```python
from build123d import *
from build123d.topology import SkipClean

# Parameters (mm, degrees)
SKETCH_1_R             = 43
SKETCH_1_R_2           = 1.75
EXTRUDE_1_DEPTH        = 3
EXTRUDE_1_2_DEPTH      = 19
EXTRUDE_1_2_DEPTH_BACK = 33
SKETCH_3_R             = 43
SKETCH_3_R_2           = 40.5
EXTRUDE_START          = -52
EXTRUDE_2_DEPTH        = 52
EXTRUDE_2_2_DEPTH      = 2.5
FILLET_1_R             = 2
SKETCH_6_W             = 12.068691
SKETCH_6_H             = 10.532676
CUT_EXTRUDE_1_DEPTH    = 3
SKETCH_7_R             = 2
CUT_EXTRUDE_2_DEPTH    = 283
SKETCH_8_R             = 2
CUT_EXTRUDE_3_DEPTH    = 10
SKETCH_9_W             = 13.11693
SKETCH_9_H             = 19.719399
CUT_EXTRUDE_4_DEPTH    = 10
SKETCH_10_W            = 7.55958
SKETCH_10_H            = 12.395118
CUT_EXTRUDE_5_DEPTH    = 61
SKETCH_11_W            = 11.880057
SKETCH_11_H            = 21.859304
CUT_EXTRUDE_6_DEPTH    = 61
SKETCH_12_R            = 4.8
CUT_EXTRUDE_7_DEPTH    = 10
SKETCH_13_R            = 4.906551
CUT_EXTRUDE_8_DEPTH    = 10


with BuildPart() as part:
    # 草图1 → Extrude 1 (new body)
    with BuildSketch(Plane.XY):
        with Locations((0, 10.35)):
            Circle(SKETCH_1_R)
        with Locations((-5, 24.315)):
            Circle(SKETCH_1_R_2, mode=Mode.SUBTRACT)
        with Locations((5, 24.315)):
            Circle(SKETCH_1_R_2, mode=Mode.SUBTRACT)
        with Locations((-5, -24.315)):
            Circle(SKETCH_1_R_2, mode=Mode.SUBTRACT)
        with Locations((5, -24.315)):
            Circle(SKETCH_1_R_2, mode=Mode.SUBTRACT)
        with BuildLine():
            Line((3.395324, 20.5), (10.5, 20.5))
            Line((10.5, 20.5), (10.5, -20.5))
            Line((10.5, -20.5), (-10.5, -20.5))
            Line((-10.5, -20.5), (-10.5, 20.5))
            Line((-10.5, 20.5), (-3.395324, 20.5))
            ThreePointArc((-3.395324, 20.5), (0, 23.895324), (3.395324, 20.5))
        make_face(mode=Mode.SUBTRACT)
        with BuildLine():
            Line((-14.5, 48.165341), (-14.5, -27.465341))
            ThreePointArc((-14.5, -27.465341), (-40.5, 10.35), (-14.5, 48.165341))
        make_face(mode=Mode.SUBTRACT)
        with BuildLine():
            Line((14.5, 48.165341), (14.5, -27.465341))
            ThreePointArc((14.5, -27.465341), (40.5, 10.35), (14.5, 48.165341))
        make_face(mode=Mode.SUBTRACT)
    extrude(amount=EXTRUDE_1_DEPTH)

    # 草图3 → Extrude 1 2 (add, two sides: drawn at the far end of the back side and taken through both)
    with SkipClean():  # the faces are left unmerged after this step: merging them gives an invalid solid
        with BuildSketch(Plane(origin=(0, 0, 0), x_dir=(-1, 0, 0), z_dir=(0, 0, -1)).offset(-EXTRUDE_1_2_DEPTH_BACK)):
            with Locations((0, 10.35)):
                Circle(SKETCH_3_R)
            with Locations((0, 10.35)):
                Circle(SKETCH_3_R_2, mode=Mode.SUBTRACT)
        extrude(amount=EXTRUDE_1_2_DEPTH + EXTRUDE_1_2_DEPTH_BACK)

    # 草图4 → Extrude 2 (add)
    with SkipClean():  # the faces are left unmerged after this step: merging them gives an invalid solid
        with BuildSketch(Plane(origin=(0, 0, -19), x_dir=(-1, 0, 0), z_dir=(0, 0, -1)).offset(EXTRUDE_START)):
            Polygon((0, 53.35), (210, 53.35), (210, -243.65), (0, -243.65), (0, -30.15), (2.5, -30.15), (2.5, -241.15), (207.5, -241.15), (207.5, 50.85), (0, 50.85), align=None)
        extrude(amount=EXTRUDE_2_DEPTH)

    # 草图5 → Extrude 2 2 (add)
    with SkipClean():  # the faces are left unmerged after this step: merging them gives an invalid solid
        with BuildSketch(Plane(origin=(0, 0, -19), x_dir=(-1, 0, 0), z_dir=(0, 0, -1))):
            with BuildLine():
                Line((2.5, -241.15), (2.5, -32.577264))
                ThreePointArc((2.5, -32.577264), (42.565682, 4.25388), (14.448183, 50.85))
                Line((14.448183, 50.85), (207.5, 50.85))
                Line((207.5, 50.85), (207.5, -241.15))
                Line((207.5, -241.15), (2.5, -241.15))
            make_face()
        extrude(amount=-EXTRUDE_2_2_DEPTH)

    # 圆角1
    fillet_1_edges = [part.edges().sort_by_distance(p)[0] for p in [
        (-207.5, 50.85, 8.25),
        (0, -243.65, 7),
        (-207.5, -241.15, 8.25),
        (-2.5, -241.15, 8.25),
        (-210, -243.65, 7),
        (-210, 53.35, 7),
    ]]
    fillet(fillet_1_edges, radius=FILLET_1_R)

    # 草图6 → 切除-拉伸1 (cut)
    with BuildSketch(Plane(origin=(0, 53.35, 0), x_dir=(1, 0, 0), z_dir=(0, 1, 0))):
        with Locations((-27.994546, 8.375655)):
            Rectangle(SKETCH_6_W, SKETCH_6_H)
    extrude(amount=-CUT_EXTRUDE_1_DEPTH, mode=Mode.SUBTRACT)

    # 草图7 → 切除-拉伸2 (cut)
    with BuildSketch(Plane(origin=(0, 0, 0), x_dir=(0, 0, -1), z_dir=(1, 0, 0))):
        with Locations(Location((-25.5, -84.801057, 0), (0, 0, 270))):
            Circle(SKETCH_7_R)
        with Locations(Location((-25.5, -190.350496, 0), (0, 0, 270))):
            Circle(SKETCH_7_R)
    extrude(amount=-CUT_EXTRUDE_2_DEPTH, mode=Mode.SUBTRACT)

    # 草图8 → 切除-拉伸3 (cut)
    with BuildSketch(Plane.XZ.offset(243.65)):
        with Locations(Location((-167.807889, 25.5, 0), (0, 0, 270))):
            Circle(SKETCH_8_R)
        with Locations(Location((-42.192111, 25.5, 0), (0, 0, 270))):
            Circle(SKETCH_8_R)
    extrude(amount=-CUT_EXTRUDE_3_DEPTH, mode=Mode.SUBTRACT)

    # 草图9 → 切除-拉伸4 (cut)
    with BuildSketch(Plane(origin=(0, 53.35, 0), x_dir=(1, 0, 0), z_dir=(0, 1, 0))):
        with Locations((-112.297275, -25.832317)):
            Rectangle(SKETCH_9_W, SKETCH_9_H)
        with BuildLine():
            Line((-92.210137, -34.22374), (-82.740067, -34.22374))
            Line((-82.740067, -34.22374), (-82.740067, -18.619532))
            ThreePointArc((-82.740067, -18.619532), (-87.475102, -14.502019), (-92.210137, -18.619532))
            Line((-92.210137, -18.619532), (-92.210137, -34.22374))
        make_face()
    extrude(amount=-CUT_EXTRUDE_4_DEPTH, mode=Mode.SUBTRACT)

    # 草图10 → 切除-拉伸5 (cut)
    with BuildSketch(Plane.ZY.offset(2.5)):
        with Locations((29.22021, 11.568763)):
            Rectangle(SKETCH_10_W, SKETCH_10_H)
    extrude(amount=CUT_EXTRUDE_5_DEPTH, mode=Mode.SUBTRACT)

    # 草图11 → 切除-拉伸6 (cut)
    with BuildSketch(Plane(origin=(0, 0, -19), x_dir=(-1, 0, 0), z_dir=(0, 0, -1))):
        with Locations((93.214773, 23.896012)):
            Rectangle(SKETCH_11_W, SKETCH_11_H)
    extrude(amount=-CUT_EXTRUDE_6_DEPTH, mode=Mode.SUBTRACT)

    # 草图12 → 切除-拉伸7 (cut)
    with BuildSketch(Plane(origin=(0, 53.35, 0), x_dir=(1, 0, 0), z_dir=(0, 1, 0))):
        with Locations(Location((-104, 6.738484, 0), (0, 0, 270))):
            Circle(SKETCH_12_R)
    extrude(amount=-CUT_EXTRUDE_7_DEPTH, mode=Mode.SUBTRACT)

    # 草图13 → 切除-拉伸8 (cut)
    with BuildSketch(Plane(origin=(0, 53.35, 0), x_dir=(1, 0, 0), z_dir=(0, 1, 0))):
        with Locations((-68.22173, -33)):
            Circle(SKETCH_13_R)
    extrude(amount=-CUT_EXTRUDE_8_DEPTH, mode=Mode.SUBTRACT)


solid = part.part
```
Work out the finished part from the listing and answer in its coordinate system (mm). A direction names the side the tool comes from. Round coordinates to 2 decimals unless told otherwise and drop trailing zeros. Loops run counter-clockwise (first coordinate to the right, second up) from the corner with the lowest first, then second, coordinate; pieces in that order, holes last. Notation, with made-up numbers: M -32.5,40 L -12.5,40 A26 ccw -12.5,72 Z; hole C -4,78 d8. An arc over 180 degrees is marked long. One line per question, with ' | ' between items.
Q1. A tool of negligible diameter and unlimited length cuts with its end or side. For faces 1 (the flat face through (0, -139, 7)), 2 (the flat face through (-106, -93, -16.5)), 3 (the flat face through (0, 29, 0)), 4 (the flat face through (-106, -243.65, 7)), from which of +Z, -Z, +X, -X, +Y, -Y can it reach the whole face along a straight path? Write none if from no direction.
Conclusion:
face 1: +Z, -Z, +X, -Y | face 2: +Z | face 3: -Z | face 4: +Z, -Z, +X, -X, -Y
Q2. The mould has two halves that part along Z. Classify faces 5 (the flat face through (0, 29, 3)), 6 (the flat face through (-113, -93, -19)), 7 (the cylindrical face through (-108.258, 52.118, -4.524)), 8 (the flat face through (-210, -93, 7)): +Z half, -Z half, draft (parallel to the pull), parting line (faces both ways), or undercut.
Conclusion:
face 5: +Z half | face 6: -Z half | face 7: undercut | face 8: draft
Q3. Each of these flat-tipped pins is pushed along its axis until it touches: pin 1 Ø4 at (x, y) = (-128, 9) entering from +Z; pin 2 Ø8.5 at (x, y) = (2, 19) entering from -Z; pin 3 Ø3 at (x, y) = (-5, 24.315) entering from -Z; pin 4 Ø4 at (y, z) = (-150.5, -1.5) entering from +X. Where does it stop, or does it pass through?
Conclusion:
pin 1: stops at z = -16.5 | pin 2: stops at z = 0 | pin 3: passes through | pin 4: stops at x = 0
Q4. Find section A-A, the plane x = -183. Give the vertices of the cut face in (y, z), then the cut area to 3 significant figures.
Conclusion:
outline: M -243.65,-19 L 53.35,-19 L 53.35,33 L 50.85,33 L 50.85,-16.5 L -241.15,-16.5 L -241.15,33 L -243.65,33 Z | area: 990 mm2
Q5. Consider line 1 along X through (y, z) = (-241.85, 25.5); line 2 along X through (y, z) = (10, -9); line 3 along X through (y, z) = (-94, 17). Determine where each line is inside the solid, lowest interval first. Write a range as from..to.
Conclusion:
line 1: x = -209.99..-169.81, -165.81..-44.19, -40.19..-0.01 | line 2: x = -210..-207.5, -43..-40.5, 40.5..43 | line 3: x = -210..-207.5, -2.5..0
